Build history of the part. All positions in model axes, mm. A direction names the side the tool comes from. Round coordinates to 2 decimals unless told otherwise and drop trailing zeros. Write each loop counter-clockwise with the first axis right and the second up, starting at its lowest first coordinate (ties: lowest second). Pieces come first, ordered by that corner, then holes. Notation, with made-up numbers: (-3.5, 15) -> (18.5, 15) arc R15 cw to (18.5, 30) -> close; hole circle Ø9 at (61, 51). An arc over 180 degrees is marked (long way). Answer as CSV lines item,"result".
from build123d import *

# Parameters (mm, degrees)
SALIENTE_EXTRUIR1_DEPTH    = 50
CORTAR_EXTRUIR1_DEPTH      = 56
CORTAR_EXTRUIR1_DEPTH_BACK = 56
CROQUIS2_W                 = 12.320508076
CROQUIS2_H                 = 30
CORTAR_EXTRUIR2_DEPTH      = 57.773277876
CORTAR_EXTRUIR2_DEPTH_BACK = 57.773277876
CROQUIS5_R                 = 10.01543576
SALIENTE_EXTRUIR2_DEPTH    = 10
CORTAR_EXTRUIR3_DEPTH      = 56
CORTAR_EXTRUIR3_DEPTH_BACK = 56
CROQUIS6_W                 = 10
CROQUIS6_H                 = 30
CROQUIS6_W_2               = 4
CORTAR_EXTRUIR4_DEPTH      = 56
CORTAR_EXTRUIR4_DEPTH_BACK = 56
CROQUIS7_R                 = 10


with BuildPart() as part:
    # Croquis1 → Saliente-Extruir1 (new, symmetric)
    with BuildSketch(Plane(origin=(0, 0, 0), x_dir=(1, 0, 0), z_dir=(0, 1, 0))):
        Polygon((-17.320508076, 0), (-8.660254038, -15), (8.660254038, -15), (17.320508076, 0), (8.660254038, 15), (-8.660254038, 15), align=None)
    extrude(amount=SALIENTE_EXTRUIR1_DEPTH, both=True)

    # Croquis2 → Cortar-Extruir1 (cut, two sides: drawn at the far end of the back side and taken through both)
    with BuildSketch(Plane.XY.offset(-CORTAR_EXTRUIR1_DEPTH_BACK)):
        with Locations((-11.160254038, -35)):
            Rectangle(CROQUIS2_W, CROQUIS2_H)
        with Locations((11.160254038, -35)):
            Rectangle(CROQUIS2_W, CROQUIS2_H)
    extrude(amount=CORTAR_EXTRUIR1_DEPTH + CORTAR_EXTRUIR1_DEPTH_BACK, mode=Mode.SUBTRACT)

    # Croquis3 → Cortar-Extruir2 (cut, two sides: drawn at the far end of the back side and taken through both)
    with BuildSketch(Plane(origin=(5, 0, 0), x_dir=(0, 0, -1), z_dir=(1, 0, 0)).offset(-CORTAR_EXTRUIR2_DEPTH_BACK)):
        with BuildLine():
            Line((-15, -35), (-15, -53.002669734))
            Line((-15, -53.002669734), (15, -53.002669734))
            Line((15, -53.002669734), (15, -35))
            ThreePointArc((15, -35), (0, -50), (-15, -35))
        make_face()
    extrude(amount=CORTAR_EXTRUIR2_DEPTH + CORTAR_EXTRUIR2_DEPTH_BACK, mode=Mode.SUBTRACT)

    # Croquis5 → Saliente-Extruir2 (add, symmetric)
    with BuildSketch(Plane(origin=(0, 0, 0), x_dir=(0, 0, -1), z_dir=(1, 0, 0))):
        with Locations((0, -35)):
            Circle(CROQUIS5_R)
    extrude(amount=SALIENTE_EXTRUIR2_DEPTH, both=True)

    # Croquis6 → Cortar-Extruir3 (cut, two sides: drawn at the far end of the back side and taken through both)
    with BuildSketch(Plane(origin=(0, 0, 0), x_dir=(0, 0, -1), z_dir=(1, 0, 0)).offset(-CORTAR_EXTRUIR3_DEPTH_BACK)):
        with Locations((0, 35)):
            Rectangle(CROQUIS6_W, CROQUIS6_H)
        with Locations((-13, 35)):
            Rectangle(CROQUIS6_W_2, CROQUIS6_H)
        with Locations((13, 35)):
            Rectangle(CROQUIS6_W_2, CROQUIS6_H)
    extrude(amount=CORTAR_EXTRUIR3_DEPTH + CORTAR_EXTRUIR3_DEPTH_BACK, mode=Mode.SUBTRACT)

    # Croquis7 → Cortar-Extruir4 (cut, two sides: drawn at the far end of the back side and taken through both)
    with BuildSketch(Plane.XY.offset(-CORTAR_EXTRUIR4_DEPTH_BACK)):
        with Locations(Location((0, 35.56624327, 0), (0, 0, 270))):
            Circle(CROQUIS7_R)
        with BuildLine():
            Line((-14.43375673, 35.56624327), (-14.43375673, 54.061973256))
            Line((-14.43375673, 54.061973256), (14.43375673, 54.061973256))
            Line((14.43375673, 54.061973256), (14.43375673, 35.56624327))
            ThreePointArc((14.43375673, 35.56624327), (0, 50), (-14.43375673, 35.56624327))
        make_face()
    extrude(amount=CORTAR_EXTRUIR4_DEPTH + CORTAR_EXTRUIR4_DEPTH_BACK, mode=Mode.SUBTRACT)


solid = part.part
1. Cut at C-C, the plane z = 1.5. Write the cut outline in (x, y).
Results found:
outline,"(-16.45, -20) -> (-5, -20) -> (-5, -25.1) -> (-10, -25.1) -> (-10, -44.9) -> (-5, -44.9) -> (-5, -49.92) -> (5, -49.92) -> (5, -44.9) -> (10, -44.9) -> (10, -25.1) -> (5, -25.1) -> (5, -20) -> (16.45, -20) -> (16.45, 20) -> (-16.45, 20) -> close"
2. Cut at D-D, the plane y = -23. Write the cut outline in (x, z), then the cut area to 3 significant figures.
Results found:
outline,"(-5, -15) -> (5, -15) -> (5, 15) -> (-5, 15) -> close"
area,"300 mm2"
3. Probe line 1 along Z through (x, y) = (-3.5, 25.5); line 2 along Y through (x, z) = (-7.5, 7); line 3 along X through (y, z) = (-41, -1.5). List the from-to ranges inside material, lowest first.
Results found:
line 1,"z = -11 to -5, 5 to 11"
line 2,"y = -42.16 to -27.84, -20 to 28.95, 42.18 to 47.9"
line 3,"x = -10 to 10"
4. Cut at A-A, the plane x = 0. Write the cut outline in (y, z).
Results found:
outline,"(-35, -15) -> (20, -15) -> (20, -11) -> (25.57, -11) -> (25.57, -5) -> (20, -5) -> (20, 5) -> (25.57, 5) -> (25.57, 11) -> (20, 11) -> (20, 15) -> (-35, 15) arc R15 ccw to start; (45.57, -11) -> (50, -11) -> (50, -5) -> (45.57, -5) -> close; (45.57, 5) -> (50, 5) -> (50, 11) -> (45.57, 11) -> close"
5. Drop flat-ended pins along their axis: pin 1 Ø5 at (x, z) = (13.5, -10) entering from +Y; pin 2 Ø12 at (x, z) = (8, 3.5) entering from +Y; pin 3 Ø12 at (x, y) = (-7, 29) entering from +Z. Give the stop position or say it passes through.
Results found:
pin 1,"stops at y = 44.91"
pin 2,"stops at y = 49.83"
pin 3,"stops at z = 11"
6. Cut at B-B, the plane y = 41.5. Write the cut outline in (x, z), then the cut area to 3 significant figures.
Results found:
outline,"(-13.16, -7.21) -> (-10.97, -11) -> (-8.05, -11) -> (-8.05, -5) -> (-13.16, -5) -> close; (-13.16, 5) -> (-8.05, 5) -> (-8.05, 11) -> (-10.97, 11) -> (-13.16, 7.21) -> close; (8.05, -11) -> (10.97, -11) -> (13.16, -7.21) -> (13.16, -5) -> (8.05, -5) -> close; (8.05, 5) -> (13.16, 5) -> (13.16, 7.21) -> (10.97, 11) -> (8.05, 11) -> close"
area,"106 mm2"
7. Mould opens along Y. For faces 4 (the flat face through (12.93, 5.712, 7.605)), 5 (the cylindrical face through (0, 50, -8)), 6 (the flat face through (5, -25, 3)), 7 (the flat face through (-10, -20, 0)) say: +Y half, -Y half, draft (parallel to the pull), parting line (faces both ways), or undercut.
Results found:
face 4,"draft"
face 5,"+Y half"
face 6,"undercut"
face 7,"undercut"
8. Which spindle directions (+Z, -Z, +X, -X, +Y, -Y) get a long thin tool onto all of the face, cutting with end or side? Do faces 1 (the flat face through (0, 25, 11)), 2 (the flat face through (0, 20, -13)), 3 (the flat face through (0, 25, -5)). Say none if no direction does.
Results found:
face 1,"+Z, +X, -X, +Y"
face 2,"-Z, +X, -X, +Y"
face 3,"+X, -X, +Y"
